Read the model definition and answer for the solid it produces. Units are mm, in the model's axes. Round coordinates to 2 decimals unless told otherwise and drop trailing zeros. Order: outer loops, then holes, each group sorted by start corner. A loop starts at its lowest first (then second) coordinate and runs counter-clockwise, first axis right, second up. Notation, with made-up numbers: M -8.5,-17.75 L 45.5,-17.75 A36 cw 45.5,19.25 Z; hole C 7.5,8.5 d7. An arc over 180 degrees is marked long. Use one line per item in the form item = value. Start each with the question number.
from build123d import *

# Parameters (mm, degrees)
F0_R     = 66
F0_R_2   = 17.5
F1_DEPTH = 37.5
F2_R     = 15
F4_DEPTH = 50
F5_R     = 1.9999


# Not quite as in the source:
# - a fillet or chamfer is up to 0.001 mm smaller than in the source, because OpenCascade refuses the exact size


with BuildPart() as f1:
    # F0 (on Top) → F1 (new body, symmetric)
    with BuildSketch(Plane.XY):
        Circle(F0_R)
        Circle(F0_R_2, mode=Mode.SUBTRACT)
    extrude(amount=F1_DEPTH, both=True)

    # F2
    f2_edges = [f1.edges().sort_by_distance(p)[0] for p in [
        (-17.5, 0, 37.5),
        (17.5, 0, 0),
        (-17.5, 0, -37.5),
        (-66, 0, -37.5),
        (66, 0, 0),
        (-66, 0, 37.5),
    ]]
    fillet(f2_edges, radius=F2_R)

    # F3 (on Top) → F4 (join)
    with BuildSketch(Plane.XY):
        with BuildLine():
            Line((2.5, -63.952634519), (-2.5, -63.952634519))
            ThreePointArc((-2.5, -63.952634519), (-4.5, -65.952634519), (-2.5, -67.952634519))
            Line((-2.5, -67.952634519), (2.5, -67.952634519))
            ThreePointArc((2.5, -67.952634519), (4.5, -65.952634519), (2.5, -63.952634519))
        make_face()
    extrude(amount=F4_DEPTH)

    # F5 (radius 2 in the source; OpenCascade refuses exactly that, so slightly less here)
    f5_edges = [f1.edges().sort_by_distance(p)[0] for p in [
        (0, -67.952635, 0),
    ]]
    fillet(f5_edges, radius=F5_R)


solid = f1.part
Item 1: Section C-C (z = 17.5) is taken. Write down the section's boundary in (x, y).
Item 2: Find the intervals of material crossed by L1, parallel to Y at x = 0, z = 11; L2, parallel to Y at x = 0, z = -13; L3, parallel to Z at x = 7, y = -46.5, in increasing order. Write a range as [from, to].
Item 3: Section B-B (y = 0) is taken. Write down the section's boundary in (x, z).
Item 4: Section A-A (z = 34.5) is taken. Write down the section's boundary in (x, y).
Item 5: For a pull along Y with two mould halves and no side action, classify faces 1 (the cylindrical face through (-4.394, -66.595, 30.997)), 2 (the cylindrical face through (60.967, -25.278, 0.315)), 3 (the flat face through (33, 1, -37.5)) as pulls with the +Y half, pulls with the -Y half, needs draft (parallel to the pull), parting line crosses it, or undercut.
Item 6: Given P1, Ø1.5, axis at y = 29, z = -27.5, coming from the -X side; P2, Ø1.5, axis at x = 51.5, y = 35, coming from the -Z side; P3, Ø4, axis at x = -51.5, z = 35, coming from the -Y side, each flat-ended and moving along its own axis, determine where each tip first touches the part or whether it passes through.
The answers:
q1.outline = M -4.5,-65.85 A2 ccw -2.5,-67.95 L 2.5,-67.95 A2 ccw 4.5,-65.85 A66 ccw long Z; hole C 0,0 d35
q2.L1 = [-67.95, -17.5], [17.5, 66]
q2.L2 = [-66, -17.5], [17.5, 66]
q2.L3 = [-37.5, 37.5]
q3.outline = M -66,-22.5 A15 ccw -51,-37.5 L -32.5,-37.5 A15 ccw -17.5,-22.5 L -17.5,22.5 A15 ccw -32.5,37.5 L -51,37.5 A15 ccw -66,22.5 Z; M 17.5,-22.5 A15 ccw 32.5,-37.5 L 51,-37.5 A15 ccw 66,-22.5 L 66,22.5 A15 ccw 51,37.5 L 32.5,37.5 A15 ccw 17.5,22.5 Z
q4.outline = C 0,0 d120; M -2.5,-67.95 L 2.5,-67.95 A2 ccw 2.5,-63.95 L -2.5,-63.95 A2 ccw Z; hole C 0,0 d47
q5.face_1 = undercut
q5.face_2 = parting line crosses it
q5.face_3 = needs draft
q6.P1 = -58.79
q6.P2 = -33.19
q6.P3 = -35.05
